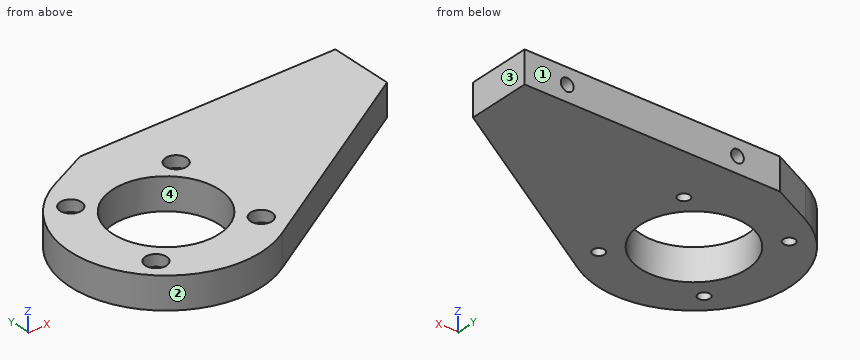
from build123d import *

# Parameters (mm, degrees)
SKETCH_R         = 25
PAD_DEPTH        = 15
HOLE_D           = 5.5
HOLE_DEPTH       = 25
HOLE_CBORE_D     = 10
HOLE_CBORE_DEPTH = 5.4
SKETCH002_R      = 3
POCKET_DEPTH     = 20


with BuildPart() as part:
    # Sketch → Pad (new body)
    with BuildSketch(Plane.XY):
        with BuildLine():
            ThreePointArc((-19.615045, 40.5), (-39.544228, -21.476825), (23.292155, -38.502929))
            Line((120, 20), (23.292155, -38.502929))
            Line((120, 50), (120, 20))
            Line((0, 50), (120, 50))
            Line((-19.615045, 40.5), (0, 50))
        make_face()
        Circle(SKETCH_R, mode=Mode.SUBTRACT)
    extrude(amount=PAD_DEPTH)

    # Hole
    with Locations(Plane.XY.offset(15)):
        with Locations((24.748737, 24.748737), (24.748737, -24.748737), (-24.748737, -24.748737), (-24.748737, 24.748737)):
            CounterBoreHole(HOLE_D / 2, HOLE_CBORE_D / 2, HOLE_CBORE_DEPTH, depth=HOLE_DEPTH)

    # Sketch002 (on Face6 of Hole) → Pocket (cut)
    with BuildSketch(Plane(origin=(0, 50, 0), x_dir=(-1, 0, 0), z_dir=(0, 1, 0))):
        with Locations((-100, 7.5)):
            Circle(SKETCH002_R)
        with Locations((-20, 7.5)):
            Circle(SKETCH002_R)
    extrude(amount=-POCKET_DEPTH, mode=Mode.SUBTRACT)


solid = part.part
The listing builds one solid part. Answer for the finished solid, in the listing's coordinates (mm). Face numbers are marked on the shaded views. Coordinates: 2 decimals unless noted, no trailing zeros. Loops run counter-clockwise (first coordinate to the right, second up) from the corner with the lowest first, then second, coordinate; pieces in that order, holes last. Notation, with made-up numbers: M 58.5,38 L 117.5,38 A8 ccw 117.5,49 Z; hole C -29.75,-37.5 d4. An arc over 180 degrees is marked long. Answer in a Markdown table with one row per item.
1) Find section C-C (z = 12.25). Determine the outline of the cut face in (x, y).
Answers below:
| item | result |
|---|---|
| outline | M -19.62,40.5 A45 ccw long 23.29,-38.5 L 120,20 L 120,50 L 0,50 Z; hole C -24.75,-24.75 d10; hole C -24.75,24.75 d10; hole C 0,0 d50; hole C 24.75,-24.75 d10; hole C 24.75,24.75 d10 |
2) Find section D-D (x = 100). Determine the outline of the cut face in (y, z).
Answers below:
| item | result |
|---|---|
| outline | M 7.9,0 L 50,0 L 50,4.5 L 30,4.5 L 30,10.5 L 50,10.5 L 50,15 L 7.9,15 Z |
3) Find section A-A (y = -3). Determine the outline of the cut face in (x, z), then the cut area to 3 significant figures.
Answers below:
| item | result |
|---|---|
| outline | M -44.9,0 L -24.82,0 L -24.82,15 L -44.9,15 Z; M 24.82,0 L 81.98,0 L 81.98,15 L 24.82,15 Z |
| area | 1,160 mm^2 |
4) Determine the mould class of the marked faces 1, 2, 3 and 4 for opening direction Y: released by +Y, released by -Y, zero draft, split by the parting line, or undercut.
Answers below:
| item | result |
|---|---|
| face 1 | released by +Y |
| face 2 | split by the parting line |
| face 3 | zero draft |
| face 4 | undercut |
5) Given pin 1 (2 mm diameter, centred on x = 18, z = 13.5, fed in from -Y); pin 2 (2 mm diameter, centred on x = -19.5, z = 12.5, fed in from +Y); pin 3 (3 mm diameter, centred on x = 20, z = 7, fed in from +Y); pin 4 (3.5 mm diameter, centred on x = -24.75, y = -24.75, fed in from -Z), each flat-ended and moving along its own axis, determine where each tip first touches the part or whether it passes through.
Answers below:
| item | result |
|---|---|
| pin 1 | y = -41.67 |
| pin 2 | y = 41.04 |
| pin 3 | y = 30 |
| pin 4 | through |
6) Find the intervals of material crossed by probe 1 along X at (y, z) = (41, 5.5); probe 2 along Z at (x, y) = (100, 38.25); probe 3 along Y at (x, z) = (-19, 12.25), in increasing order.
Answers below:
| item | result |
|---|---|
| probe 1 | -18.58 to 17.76, 22.24 to 97.76, 102.24 to 120 |
| probe 2 | 0 to 4.5, 10.5 to 15 |
| probe 3 | -40.79 to -16.25, 16.25 to 40.8 |
7) Find section B-B (x = 14.5). Determine the outline of the cut face in (y, z), then the cut area to 3 significant figures.
Answers below:
| item | result |
|---|---|
| outline | M -42.6,0 L -20.37,0 L -20.37,15 L -42.6,15 Z; M 20.37,0 L 50,0 L 50,15 L 20.37,15 Z |
| area | 778 mm^2 |
